from build123d import *

# Parameters (mm, degrees)
SKETCH1_R           = 1.75
SKETCH1_R_2         = 10
BOSS_EXTRUDE1_DEPTH = 3
FILLET1_R           = 10


with BuildPart() as part:
    # Sketch1 → Boss-Extrude1 (new body)
    with BuildSketch(Plane.XY):
        with BuildLine():
            Line((-39.9, -10.928932188), (-39.9, 10.928932188))
            ThreePointArc((-39.9, 10.928932188), (-39.519397663, 12.84234935), (-38.435533906, 14.464466094))
            Line((-38.435533906, 14.464466094), (-36.364466094, 16.535533906))
            ThreePointArc((-36.364466094, 16.535533906), (-34.74234935, 17.619397663), (-32.828932188, 18))
            Line((-32.828932188, 18), (32.828932188, 18))
            ThreePointArc((32.828932188, 18), (34.74234935, 17.619397663), (36.364466094, 16.535533906))
            Line((36.364466094, 16.535533906), (38.435533906, 14.464466094))
            ThreePointArc((38.435533906, 14.464466094), (39.519397663, 12.84234935), (39.9, 10.928932188))
            Line((39.9, 10.928932188), (39.9, -10.928932188))
            ThreePointArc((39.9, -10.928932188), (39.519397663, -12.84234935), (38.435533906, -14.464466094))
            Line((38.435533906, -14.464466094), (34.9, -18))
            Line((34.9, -18), (8.1, -18))
            Line((8.1, -18), (-8.1, -18))
            Line((-8.1, -18), (-34.9, -18))
            Line((-34.9, -18), (-38.435533906, -14.464466094))
            ThreePointArc((-38.435533906, -14.464466094), (-39.519397663, -12.84234935), (-39.9, -10.928932188))
        make_face()
        with Locations((-32.828932188, 13)):
            Circle(SKETCH1_R, mode=Mode.SUBTRACT)
        with Locations((-33, -13.5)):
            Circle(SKETCH1_R, mode=Mode.SUBTRACT)
        with Locations(Location((33, -13.5, 0), (0, 0, 180))):
            Circle(SKETCH1_R, mode=Mode.SUBTRACT)
        with Locations(Location((32.828932188, 13, 0), (0, 0, 180))):
            Circle(SKETCH1_R, mode=Mode.SUBTRACT)
        Circle(SKETCH1_R_2, mode=Mode.SUBTRACT)
    extrude(amount=BOSS_EXTRUDE1_DEPTH)

    # Fillet1
    fillet1_edges = [part.edges().sort_by_distance(p)[0] for p in [
        (34.9, -18, 1.5),
        (-34.9, -18, 1.5),
    ]]
    fillet(fillet1_edges, radius=FILLET1_R)


solid = part.part
Verification items for the finished model (mm, model axes). Give positions to 0.01 mm unless a question says otherwise; leave off trailing zeros. Write each loop counter-clockwise with the first axis right and the second up, starting at its lowest first coordinate (ties: lowest second). Pieces come first, ordered by that corner, then holes. Notation, with made-up numbers: (57, 73.25) -> (70, 73.25) arc R20 ccw to (70, 78.25) -> close; hole circle Ø2 at (-37.5, 5.5). An arc over 180 degrees is marked (long way). Use CSV: the item, a comma, the result in double quotes.
(1) Release check for a two-part mould opening along Y. For faces 1 (the cylindrical face through (34.1, 11.8, 1.5)), 2 (the flat face through (-37.4, 15.5, 1.5)), 3 (the cylindrical face through (34.53, -17.26, 1.52)) record: +Y half, -Y half, draft (parallel to the pull), parting line (faces both ways), or undercut.
Derived:
face 1,"undercut"
face 2,"+Y half"
face 3,"-Y half"
(2) Sectioned sample at C-C (z = 1.4). Record the cut outline in (x, y).
Derived:
outline,"(-39.9, -10.93) arc R5 ccw to (-38.44, -14.46) -> (-37.83, -15.07) arc R10 ccw to (-30.76, -18) -> (30.76, -18) arc R10 ccw to (37.83, -15.07) -> (38.44, -14.46) arc R5 ccw to (39.9, -10.93) -> (39.9, 10.93) arc R5 ccw to (38.44, 14.46) -> (36.36, 16.54) arc R5 ccw to (32.83, 18) -> (-32.83, 18) arc R5 ccw to (-36.36, 16.54) -> (-38.44, 14.46) arc R5 ccw to (-39.9, 10.93) -> close; hole circle Ø3.5 at (-33, -13.5); hole circle Ø3.5 at (-32.83, 13); hole circle Ø20 at (0, 0); hole circle Ø3.5 at (32.83, 13); hole circle Ø3.5 at (33, -13.5)"
(3) Sectioned sample at D-D (y = 13). Record the cut outline in (x, z), plus the area to 3 significant figures.
Derived:
outline,"(-39.45, 0) -> (-34.58, 0) -> (-34.58, 3) -> (-39.45, 3) -> close; (-31.08, 0) -> (31.08, 0) -> (31.08, 3) -> (-31.08, 3) -> close; (34.58, 0) -> (39.45, 0) -> (39.45, 3) -> (34.58, 3) -> close"
area,"216 mm^2"
(4) Material ranges on L1, parallel to Y at x = -33, z = 1.7; L2, parallel to Y at x = 31.5, z = 2.55; L3, parallel to X at y = -11, z = 1.15, recorded low to high.
Derived:
L1,"y = -17.75 to -15.25, -11.75 to 11.26, 14.74 to 18"
L2,"y = -17.97 to -14.4, -12.6 to 11.86, 14.14 to 18"
L3,"x = -39.9 to 39.9"
(5) Sectioned sample at B-B (y = 0). Record the cut outline in (x, z).
Derived:
outline,"(-39.9, 0) -> (-10, 0) -> (-10, 3) -> (-39.9, 3) -> close; (10, 0) -> (39.9, 0) -> (39.9, 3) -> (10, 3) -> close"
(6) Sectioned sample at A-A (x = 0). Record the cut outline in (y, z).
Derived:
outline,"(-18, 0) -> (-10, 0) -> (-10, 3) -> (-18, 3) -> close; (10, 0) -> (18, 0) -> (18, 3) -> (10, 3) -> close"
